Geometry: final body of the model. Coordinates: model frame, mm. A direction names the side the tool comes from. Give positions to 0.01 mm unless a question says otherwise; leave off trailing zeros. Loops run counter-clockwise (first coordinate to the right, second up) from the corner with the lowest first, then second, coordinate; pieces in that order, holes last. Notation, with made-up numbers: (-16.75, -15) -> (12.25, -15) arc R33 ccw to (12.25, 13) -> close; hole circle Ø1 at (74.25, 85). An arc over 180 degrees is marked (long way). One line per item, written item: value. Start each with the question number.
from build123d import *

# Parameters (mm, degrees)
SCHIZZO1_R                   = 4
ESTRUSIONE_ESTRUSIONE1_DEPTH = 35
SMUSSO1_SIZE                 = 1
SCHIZZO6_R                   = 6.5
ESTRUSIONE_ESTRUSIONE3_DEPTH = 8
TAGLIO_ESTRUSIONE3_DEPTH     = 6
SCHIZZO8_R                   = 3.464101615
TAGLIO_ESTRUSIONE4_DEPTH     = 1
TAGLIO_ESTRUSIONE4_TAPER     = 45
RACCORDO1_R                  = 0.5
SCHIZZO9_R                   = 8
SCHIZZO9_R_2                 = 6.5
ESTRUSIONE_ESTRUSIONE4_DEPTH = 1
RACCORDO2_R                  = 0.1


with BuildPart() as part:
    # Schizzo1 → Estrusione-Estrusione1 (new body)
    with BuildSketch(Plane.XY):
        Circle(SCHIZZO1_R)
    extrude(amount=ESTRUSIONE_ESTRUSIONE1_DEPTH)

    # Smusso1
    smusso1_edges = [part.edges().sort_by_distance(p)[0] for p in [
        (-4, 0, 0),
    ]]
    chamfer(smusso1_edges, length=SMUSSO1_SIZE)

    # Schizzo6 → Estrusione-Estrusione3 (add)
    with BuildSketch(Plane.XY.offset(35)):
        Circle(SCHIZZO6_R)
    extrude(amount=ESTRUSIONE_ESTRUSIONE3_DEPTH)

    # Schizzo7 → Taglio-Estrusione3 (cut)
    with BuildSketch(Plane.XY.offset(43)):
        Polygon((1.732050808, 3), (-1.732050808, 3), (-3.464101615, 0), (-1.732050808, -3), (1.732050808, -3), (3.464101615, 0), align=None)
    extrude(amount=-TAGLIO_ESTRUSIONE3_DEPTH, mode=Mode.SUBTRACT)

    # Schizzo8 → Taglio-Estrusione4 (cut)
    with BuildSketch(Plane.XY.offset(43)):
        Circle(SCHIZZO8_R)
    extrude(amount=-TAGLIO_ESTRUSIONE4_DEPTH, taper=TAGLIO_ESTRUSIONE4_TAPER, mode=Mode.SUBTRACT)

    # Raccordo1
    raccordo1_edges = [part.edges().sort_by_distance(p)[0] for p in [
        (-6.5, 0, 43),
    ]]
    fillet(raccordo1_edges, radius=RACCORDO1_R)

    # Schizzo9 → Estrusione-Estrusione4 (add)
    with BuildSketch(Plane(origin=(0, 0, 35), x_dir=(-1, 0, 0), z_dir=(0, 0, -1))):
        Circle(SCHIZZO9_R)
        Circle(SCHIZZO9_R_2, mode=Mode.SUBTRACT)
    extrude(amount=-ESTRUSIONE_ESTRUSIONE4_DEPTH)

    # Raccordo2
    raccordo2_edges = [part.edges().sort_by_distance(p)[0] for p in [
        (-6.5, 0, 36),
        (8, 0, 36),
        (8, 0, 35),
    ]]
    fillet(raccordo2_edges, radius=RACCORDO2_R)


solid = part.part
Item 1: Section C-C, the plane z = 18. Output: boundary loops of the cut face in (x, y), then the cut area to 3 significant figures.
Item 2: Section A-A, the plane x = 0. Output: boundary loops of the cut face in (y, z), then the cut area to 3 significant figures.
Item 3: Section B-B, the plane z = 36.5. Output: boundary loops of the cut face in (x, y), then the cut area to 3 significant figures.
Item 4: Mould query, pull axis Y, two halves, no side actions, for faces 1 (the face through (0, -3, 40)), 2 (the face through (5, -5, 36)), 3 (the face through (1.73, -7.81, 35.49)). Classes: pulls with the +Y half, pulls with the -Y half, needs draft (parallel to the pull), parting line crosses it, or undercut.
Item 5: Pin query (flat end, axial travel): pin 1 (3 mm diameter, centred on x = -2, y = 6, fed in from -Z); pin 2 (4 mm diameter, centred on x = 0.5, z = 39.5, fed in from -Y); pin 3 (1.8 mm diameter, centred on x = 0.5, y = 1.5, fed in from +Z). Return the tip coordinate at first contact, or that it passes through.
Item 6: Access query for faces 4 (the face through (3, -3, 43)), 5 (the face through (0, 3, 40)), 6 (the face through (4, 2, 35)). Directions: +Z, -Z, +X, -X, +Y, -Y. A direction counts if a zero-diameter tool reaches every point of the face in a straight line with its end or side. Return the directions, or none.
Item 7: Ray query, line 1 along Z through (x, y) = (-5.5, -1.5); line 2 along Z through (x, y) = (4.25, 5); line 3 along Y through (x, z) = (-0.75, 38). Return the intervals inside material, ascending. Write a range as [from, to].
Geometry check:
1. outline: circle Ø8 at (0, 0)
1. area: 50.3 mm2
2. outline: (-8, 35.1) arc R0.1 ccw to (-7.9, 35) -> (-4, 35) -> (-4, 1) -> (-3, 0) -> (3, 0) -> (4, 1) -> (4, 35) -> (7.9, 35) arc R0.1 ccw to (8, 35.1) -> (8, 35.9) arc R0.1 ccw to (7.9, 36) -> (6.6, 36) arc R0.1 cw to (6.5, 36.1) -> (6.5, 42.5) arc R0.5 ccw to (6, 43) -> (3.46, 43) -> (3, 42.54) -> (3, 37) -> (-3, 37) -> (-3, 42.54) -> (-3.46, 43) -> (-6, 43) arc R0.5 ccw to (-6.5, 42.5) -> (-6.5, 36.1) arc R0.1 cw to (-6.6, 36) -> (-7.9, 36) arc R0.1 ccw to (-8, 35.9) -> close
2. area: 350 mm2
3. outline: circle Ø13 at (0, 0)
3. area: 133 mm2
4. face 1: undercut
4. face 2: needs draft
4. face 3: parting line crosses it
5. pin 1: stops at z = 35
5. pin 2: stops at y = -6.5
5. pin 3: stops at z = 37
6. face 4: +Z, +X, -X, +Y, -Y
6. face 5: +Z
6. face 6: -Z
7. line 1: z = [35, 43]
7. line 2: z = [35, 36.01]
7. line 3: y = [-6.46, -3], [3, 6.46]
